The model under review builds one solid part; all positions refer to its coordinate system, in mm. A direction names the side the tool comes from. Round coordinates to 2 decimals unless told otherwise and drop trailing zeros. Order: outer loops, then holes, each group sorted by start corner. A loop starts at its lowest first (then second) coordinate and runs counter-clockwise, first axis right, second up. Notation, with made-up numbers: (25.5, -24.75) -> (30.5, -24.75) arc R21 cw to (30.5, 7.25) -> close; hole circle Ø4 at (-13.75, 44). An arc over 180 degrees is marked (long way). Use a Markdown table: item, result. Add a question column.
```python
from build123d import *

# Parameters (mm, degrees)
CROQUIS1_W              = 350
CROQUIS1_H              = 60
SALIENTE_EXTRUIR1_DEPTH = 6
CROQUIS2_R              = 6
CROQUIS2_R_2            = 1.25
CORTAR_EXTRUIR1_DEPTH   = 7
CROQUIS3_R              = 6
CROQUIS3_R_2            = 1.5
CROQUIS3_R_3            = 2.5
CORTAR_EXTRUIR2_DEPTH   = 7
CROQUIS5_R              = 19.5
CORTAR_EXTRUIR4_DEPTH   = 2
CROQUIS7_R              = 4
CORTAR_EXTRUIR5_DEPTH   = 5


with BuildPart() as part:
    # Croquis1 → Saliente-Extruir1 (new body)
    with BuildSketch(Plane.XY):
        with Locations((-175, -30)):
            Rectangle(CROQUIS1_W, CROQUIS1_H)
    extrude(amount=SALIENTE_EXTRUIR1_DEPTH)

    # Croquis2 → Cortar-Extruir1 (cut, through all)
    with BuildSketch(Plane.XY.offset(6)):
        with Locations((-327.5, -22.5)):
            Circle(CROQUIS2_R)
        with Locations((-22.5, -22.5)):
            Circle(CROQUIS2_R)
        with Locations((-314.595301243, -9.595301243)):
            Circle(CROQUIS2_R_2)
        with Locations((-340.404698757, -35.404698757)):
            Circle(CROQUIS2_R_2)
        with Locations((-35.404698757, -9.595301243)):
            Circle(CROQUIS2_R_2)
        with Locations((-9.595301243, -35.404698757)):
            Circle(CROQUIS2_R_2)
    extrude(amount=-CORTAR_EXTRUIR1_DEPTH, mode=Mode.SUBTRACT)

    # Croquis3 → Cortar-Extruir2 (cut, through all)
    with BuildSketch(Plane.XY.offset(6)):
        with Locations((-175, -28)):
            Circle(CROQUIS3_R)
        with Locations((-190.5, -12.5)):
            Circle(CROQUIS3_R_2)
        with Locations((-159.5, -12.5)):
            Circle(CROQUIS3_R_2)
        with Locations((-190.5, -43.5)):
            Circle(CROQUIS3_R_2)
        with Locations((-151.45, -51.55)):
            Circle(CROQUIS3_R_3)
        with Locations((-198.55, -51.55)):
            Circle(CROQUIS3_R_3)
        with Locations((-159.5, -43.5)):
            Circle(CROQUIS3_R_2)
        with Locations((-151.45, -4.45)):
            Circle(CROQUIS3_R_3)
        with Locations((-198.55, -4.45)):
            Circle(CROQUIS3_R_3)
    extrude(amount=-CORTAR_EXTRUIR2_DEPTH, mode=Mode.SUBTRACT)

    # Croquis5 → Cortar-Extruir4 (cut)
    with BuildSketch(Plane.XY.offset(6)):
        with Locations((-175, -28)):
            Circle(CROQUIS5_R)
        with BuildLine():
            Line((-292, 0), (-252, 0))
            Line((-252, 0), (-252, -32))
            ThreePointArc((-252, -32), (-254.343145751, -37.656854249), (-260, -40))
            Line((-260, -40), (-284, -40))
            ThreePointArc((-284, -40), (-289.656854249, -37.656854249), (-292, -32))
            Line((-292, -32), (-292, 0))
        make_face()
        with BuildLine():
            Line((-98, 0), (-58, 0))
            Line((-58, 0), (-58, -32))
            ThreePointArc((-58, -32), (-60.343145751, -37.656854249), (-66, -40))
            Line((-66, -40), (-90, -40))
            ThreePointArc((-90, -40), (-95.656854249, -37.656854249), (-98, -32))
            Line((-98, -32), (-98, 0))
        make_face()
    extrude(amount=-CORTAR_EXTRUIR4_DEPTH, mode=Mode.SUBTRACT)

    # Croquis7 → Cortar-Extruir5 (cut, through all)
    with BuildSketch(Plane.XY.offset(4)):
        with Locations((-272, -20)):
            Circle(CROQUIS7_R)
        with Locations((-78, -20)):
            Circle(CROQUIS7_R)
    extrude(amount=-CORTAR_EXTRUIR5_DEPTH, mode=Mode.SUBTRACT)


solid = part.part
```
Q1. For faces 5 (the face through (-181, -28, 2)), 6 (the face through (-289.594, -37.719, 5.014)), 7 (the face through (-171, -23, 4)), list the 3-axis set-ups (+Z, -Z, +X, -X, +Y, -Y) from which the entire face can be reached by the end or side of a thin tool; tool diameter is ignored.
Q2. Draft analysis for pull direction X (two halves, no side actions). For faces 1 (the face through (-350, -30, 3)), 2 (the face through (-177, -50, 6)), 3 (the face through (-254.281, -37.594, 5.014)), 4 (the face through (-276, -20, 2)), state which applies: released by +X, released by -X, zero draft, split by the parting line, or undercut.
Q3. For pin 1 (10.5 mm diameter, centred on x = -78, y = -20, fed in from +Z); pin 2 (3 mm diameter, centred on x = -151.45, y = -51.55, fed in from +Z), all flat-tipped, find the tip position at first contact; note any pin that passes through.
Q4. Add section C-C, the plane z = 1.75. Give the number of separate pieces and of enclosed holes in the cut face, then the cut area to 3 significant figures.
Q5. Add section D-D, the plane x = -23. Give the boundary of the cut face in (y, z).
Q6. Add section A-A, the plane x = -175. Give the boundary of the cut face in (y, z).
Q7. To check wall thickness, follow line 1 along Y through (x, z) = (-198.55, 1.6); line 2 along Y through (x, z) = (-159.5, 2.6); line 3 along X through (y, z) = (-20.5, 4.5). State the ranges of each line that lie inside material, in increasing order.
Q8. Add section B-B, the plane x = -263.5. Give the boundary of the cut face in (y, z).
Return value:
| question | item | result |
|---|---|---|
| 1 | face 5 | +Z, -Z |
| 1 | face 6 | +Z, +Y |
| 1 | face 7 | +Z |
| 2 | face 1 | released by -X |
| 2 | face 2 | zero draft |
| 2 | face 3 | undercut |
| 2 | face 4 | undercut |
| 3 | pin 1 | z = 4 |
| 3 | pin 2 | through |
| 4 | separate pieces | 1 |
| 4 | enclosed holes | 17 |
| 4 | area | 20,400 mm² |
| 5 | outline | (-60, 0) -> (-28.48, 0) -> (-28.48, 6) -> (-60, 6) -> close; (-16.52, 0) -> (0, 0) -> (0, 6) -> (-16.52, 6) -> close |
| 6 | outline | (-60, 0) -> (-34, 0) -> (-34, 4) -> (-47.5, 4) -> (-47.5, 6) -> (-60, 6) -> close; (-22, 0) -> (0, 0) -> (0, 6) -> (-8.5, 6) -> (-8.5, 4) -> (-22, 4) -> close |
| 7 | line 1 | -60 to -54.05, -49.05 to -6.95, -1.95 to 0 |
| 7 | line 2 | -60 to -45, -42 to -14, -11 to 0 |
| 7 | line 3 | -350 to -333.16, -321.84 to -292, -252 to -193, -157 to -98, -58 to -28.16, -16.84 to 0 |
| 8 | outline | (-60, 0) -> (0, 0) -> (0, 4) -> (-40, 4) -> (-40, 6) -> (-60, 6) -> close |
